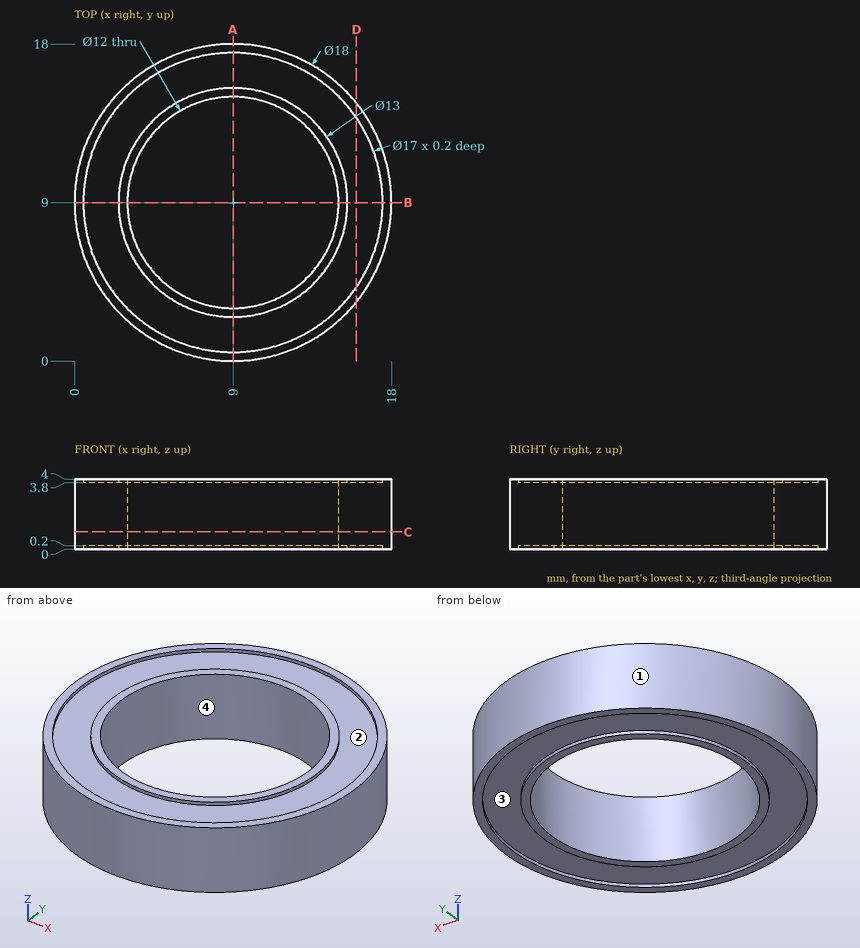
Geometry: see drawing. Coordinates: mm, zero at the bounding-box minimum. A direction names the side the tool comes from. Coordinates: 2 decimals unless noted, no trailing zeros. Loops run counter-clockwise (first coordinate to the right, second up) from the corner with the lowest first, then second, coordinate; pieces in that order, holes last. Notation, with made-up numbers: M 61,3 L 71,3 A23 ccw 71,18 Z; hole C 57.25,8 d5. An arc over 180 degrees is marked long. Answer in a Markdown table with one row per item.
Q1. Set-up query: the marked faces 3 and 4. Return all of +Z, -Z, +X, -X, +Y, -Y with unobstructed straight access to the full face (end or side cutting, diameter ignored); none if empty.
Answers below:
| item | result |
|---|---|
| face 3 | -Z |
| face 4 | +Z, -Z |
Q2. Ray query, probe 1 along Y at (x, z) = (9, 0.1); probe 2 along Y at (x, z) = (9, 0.9); probe 3 along Z at (x, y) = (6, 2.25). Return the intervals inside material, ascending. Write a range as from..to.
Answers below:
| item | result |
|---|---|
| probe 1 | y = 0..0.5, 2.5..3, 15..15.5, 17.5..18 |
| probe 2 | y = 0..3, 15..18 |
| probe 3 | z = 0.2..3.8 |
Q3. Section C-C on z = 1. Return the cut outline in (x, y).
Answers below:
| item | result |
|---|---|
| outline | C 9,9 d18; hole C 9,9 d12 |
Q4. Section D-D on x = 16. Return the cut outline in (y, z).
Answers below:
| item | result |
|---|---|
| outline | M 3.34,0 L 4.18,0 L 4.18,0.2 L 13.82,0.2 L 13.82,0 L 14.66,0 L 14.66,4 L 13.82,4 L 13.82,3.8 L 4.18,3.8 L 4.18,4 L 3.34,4 Z |
Q5. Section A-A on x = 9. Return the cut outline in (y, z), plus the area to 3 significant figures.
Answers below:
| item | result |
|---|---|
| outline | M 0,0 L 0.5,0 L 0.5,0.2 L 2.5,0.2 L 2.5,0 L 3,0 L 3,4 L 2.5,4 L 2.5,3.8 L 0.5,3.8 L 0.5,4 L 0,4 Z; M 15,0 L 15.5,0 L 15.5,0.2 L 17.5,0.2 L 17.5,0 L 18,0 L 18,4 L 17.5,4 L 17.5,3.8 L 15.5,3.8 L 15.5,4 L 15,4 Z |
| area | 22.4 mm^2 |
Q6. Draft query along Y for the marked faces 1 and 2. Return one class per face: pulls with the +Y half, pulls with the -Y half, needs draft (parallel to the pull), parting line crosses it, or undercut.
Answers below:
| item | result |
|---|---|
| face 1 | parting line crosses it |
| face 2 | undercut |
Q7. First-contact query: pin 1 (5 mm diameter, centred on x = 9.5, y = 12.5, fed in from -Z); pin 2 (2 mm diameter, centred on x = 12.5, z = 2.5, fed in from -Y); pin 3 (1 mm diameter, centred on x = 12.5, y = 9, fed in from +Z); pin 4 (1.5 mm diameter, centred on y = 10, z = 2.5, fed in from -X). Flat tips, straight axial feed; report the tip coordinate or a pass-through.
Answers below:
| item | result |
|---|---|
| pin 1 | stops at z = 0 |
| pin 2 | stops at y = 0.35 |
| pin 3 | passes through |
| pin 4 | stops at x = 0 |
